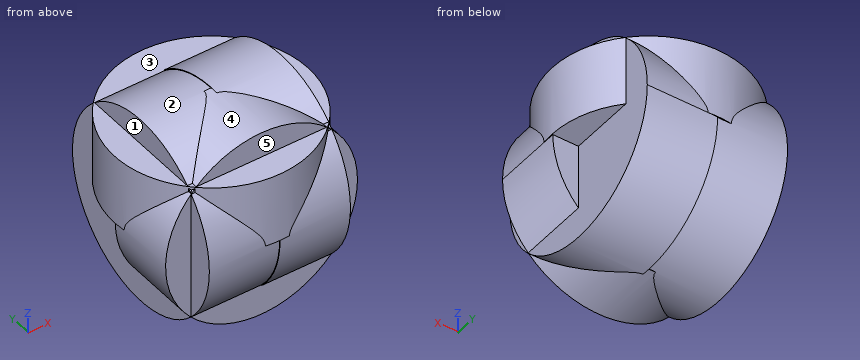
```python
from build123d import *

# Parameters (mm, degrees)
F0_R      = 69.29858
F1_DEPTH  = 50.8
F2_R      = 69.381637
F3_DEPTH  = 50.8
F4_R      = 69.544385
F5_DEPTH  = 50.8
F6_R      = 69.112883
F7_DEPTH  = 50.8
F8_R      = 69.874838
F9_DEPTH  = 50.8
F10_R     = 69.061616
F11_DEPTH = 50.8


with BuildPart() as f1:
    # F0 (on Front) → F1 (new body)
    with BuildSketch(Plane.XZ):
        Circle(F0_R)
    extrude(amount=F1_DEPTH)

    # F2 (on Top) → F3 (join)
    with BuildSketch(Plane.XY):
        Circle(F2_R)
    extrude(amount=F3_DEPTH)

    # F4 (on Right) → F5 (join)
    with BuildSketch(Plane.YZ):
        Circle(F4_R)
    extrude(amount=F5_DEPTH)

    # F6 (on Right) → F7 (join)
    with BuildSketch(Plane.YZ):
        Circle(F6_R)
    extrude(amount=-F7_DEPTH)

    # F8 (on Top) → F9 (join)
    with BuildSketch(Plane.XY):
        Circle(F8_R)
    extrude(amount=F9_DEPTH)

    # F10 (on Front) → F11 (join)
    with BuildSketch(Plane.XZ):
        Circle(F10_R)
    extrude(amount=F11_DEPTH)


solid = f1.part
```
Geometry: final body of the model. Coordinates: model frame, mm. Face numbers are marked on the shaded views. A direction names the side the tool comes from. Coordinates: 2 decimals unless noted, no trailing zeros. Loops run counter-clockwise (first coordinate to the right, second up) from the corner with the lowest first, then second, coordinate; pieces in that order, holes last. Notation, with made-up numbers: (54.5, 39.25) -> (97.5, 39.25) arc R15 cw to (97.5, 61.25) -> close; hole circle Ø7 at (-34.5, -21). An arc over 180 degrees is marked (long way). Use a Markdown table: item, result. Add a question column.
(1) Section query C-C, the plane x = -60. Return loops of the section in (y, z), plus the area to 3 significant figures.
(2) Access query for the marked faces 1, 2, 3, 4 and 5. Directions: +Z, -Z, +X, -X, +Y, -Y. A direction counts if a zero-diameter tool reaches every point of the face in a straight line with its end or side. Return the directions, or none.
(3) Section query B-B, the plane z = 5. Return loops of the section in (x, y).
(4) Pin query (flat end, axial travel): pin 1 Ø15.5 at (x, y) = (58, 6.5) entering from -Z; pin 2 Ø12 at (y, z) = (-26.5, 39.5) entering from -X; pin 3 Ø5.5 at (x, z) = (7, 64.5) entering from -Y. Return the tip coordinate at first contact, or that it passes through.
(5) Section query A-A, the plane y = 38.5. Return loops of the section in (x, z).
(6) Section query D-D, the plane y = 53. Return loops of the section in (x, z).
(7) Line query: line 1 along X through (y, z) = (41.5, -53.5); line 2 along Y through (x, z) = (62, -6); line 3 along Y through (x, z) = (41.5, 0). Output: solid intervals per line, ascending.
Answer:
| question | item | result |
|---|---|---|
| 1 | outline | (-50.8, -34.67) -> (0, -34.67) -> (0, 0) -> (35.81, 0) -> (35.81, 50.8) -> (-35.81, 50.8) -> (-35.81, 34.67) -> (-50.8, 34.67) -> close |
| 1 | area | 5,920 mm^2 |
| 2 | face 1 | +Z, -X, +Y, -Y |
| 2 | face 2 | +Z, -X |
| 2 | face 3 | +Z |
| 2 | face 4 | +Z, -Y |
| 2 | face 5 | +Z, +X, -X, -Y |
| 3 | outline | (-69.12, -50.8) -> (-50.8, -50.8) -> (-50.8, -68.93) -> (-11.44, -68.93) arc R69.87 ccw to (8.43, -69.36) -> (50.8, -69.36) -> (50.8, -50.8) -> (69.12, -50.8) -> (69.12, -10.26) arc R69.87 ccw to (50.8, 47.98) -> (50.8, 69.36) -> (8.43, 69.36) arc R69.87 ccw to (-11.44, 68.93) -> (-50.8, 68.93) -> (-50.8, 47.98) arc R69.87 ccw to (-69.12, -10.26) -> close |
| 4 | pin 1 | stops at z = -69.45 |
| 4 | pin 2 | stops at x = -66.8 |
| 4 | pin 3 | stops at y = -50.8 |
| 5 | outline | (-58.31, 0) -> (-50.8, 0) -> (-50.8, -57.4) -> (0, -57.4) -> (0, -57.92) -> (50.8, -57.92) -> (50.8, 0) -> (58.31, 0) -> (58.31, 50.8) -> (50.8, 50.8) -> (50.8, 57.92) -> (0, 57.92) -> (0, 57.4) -> (-50.8, 57.4) -> (-50.8, 50.8) -> (-58.31, 50.8) -> close |
| 6 | outline | (-50.8, -44.36) -> (0, -44.36) -> (0, -45.03) -> (50.8, -45.03) -> (50.8, 45.03) -> (45.54, 45.03) -> (45.54, 50.8) -> (-45.54, 50.8) -> (-45.54, 44.36) -> (-50.8, 44.36) -> close |
| 7 | line 1 | x = -50.8 to 50.8 |
| 7 | line 2 | y = -50.8 to 0 |
| 7 | line 3 | y = -69.54 to 69.54 |
